Check sheet for the modelled part. Datum: model origin and axes. Units: mm. A direction names the side the tool comes from. Coordinates: 2 decimals unless noted, no trailing zeros. Loops run counter-clockwise (first coordinate to the right, second up) from the corner with the lowest first, then second, coordinate; pieces in that order, holes last. Notation, with made-up numbers: M 81.5,48 L 85.5,48 A13 cw 85.5,60 Z; hole C 58.25,27.5 d8. An arc over 180 degrees is marked long. Answer in a Markdown table with one row per item. Add a question column.
```python
from build123d import *

# Parameters (mm, degrees)
F0_R     = 14
F0_R_2   = 1.1
F1_DEPTH = 8
F3_DEPTH = 8.001
F6_R     = 0.875
F7_DEPTH = 19.125355653


# Not quite as in the source:
# - a pattern or mirror of a feature is missing from the dataset's text; its kind, count and spacing are read off the source's solid


with BuildPart() as f1:
    # F0 (on Front) → F1 (new body)
    with BuildSketch(Plane.XZ):
        Circle(F0_R)
        with Locations((-8.6602540378, -5)):
            Circle(F0_R_2, mode=Mode.SUBTRACT)
        with Locations((8.6602540378, -5)):
            Circle(F0_R_2, mode=Mode.SUBTRACT)
        with Locations((0, 10)):
            Circle(F0_R_2, mode=Mode.SUBTRACT)
    extrude(amount=F1_DEPTH)

    # F2 (on face) → F3 (cut, through all)
    with BuildSketch(Plane.XZ.offset(8)):
        with BuildLine():
            Line((-1.5, -1.3228756555), (1.5, -1.3228756555))
            ThreePointArc((1.5, -1.3228756555), (0, 2), (-1.5, -1.3228756555))
        make_face()
    extrude(amount=-F3_DEPTH, mode=Mode.SUBTRACT)

    # F6 (on line) → F7 (cut, through all)
    with BuildSketch(Plane(origin=(0, 0, 0), x_dir=(0, 1, 0), z_dir=(0.8660254038, 0, -0.5))):
        with Locations((-4, 0)):
            Circle(F6_R)
    f7 = extrude(amount=-F7_DEPTH, mode=Mode.SUBTRACT)

    # F7_copies: F7 across plane
    add(f7.mirror(Plane(origin=(1.9e-05, 0, 0), x_dir=(-1e-06, 0, 1), z_dir=(1, 0, 1e-06))), mode=Mode.SUBTRACT)


solid = f1.part
```
Q1. Cross-section at C-C (z = -5). Record the cut outline in (x, y).
Q2. Thickness scan on L1, parallel to X at y = -6.5, z = -5.5; L2, parallel to X at y = -6.5, z = -5.25; L3, parallel to Z at x = 9.25, y = -0.5. Record the ranges inside material, lowest first.
Q3. Go/stop test with flat-tipped pins: pin 1 (1.8 mm diameter, centred on x = 0, z = 10, fed in from -Y); pin 2 (3 mm diameter, centred on y = -2, z = 9, fed in from +X); pin 3 (4 mm diameter, centred on y = -6, z = -6, fed in from +X); pin 4 (1 mm diameter, centred on y = -4.5, z = -6, fed in from +X). Record where each tip stops, or that it passes through.
Q4. Mould release check, pull along X, two halves, no side actions. Record for faces 1 (the face through (0, -4, 2)), 2 (the face through (0, 0, -3)), 3 (the face through (12.932, -3.944, -5.362)), 4 (the face through (7.56, -3.94, -4.95)): released by +X, released by -X, zero draft, split by the parting line, or undercut.
Q5. Access from +Z, -Z, +X, -X, +Y, -Y to the whole of each face (thin tool, end or side, straight path). Record for faces 5 (the face through (6.636, -3.165, 4.135)), 6 (the face through (0, -4, -1.323)).
Q6. Cross-section at B-B (y = -3.75). Record the cut outline in (x, z), plus the area to 3 significant figures.
Q7. Cross-section at D-D (z = 10.75). Record the cut outline in (x, y), plus the area to 3 significant figures.
Q8. Cross-section at A-A (x = 0). Record the cut outline in (y, z).
Answer key:
| question | item | result |
|---|---|---|
| 1 | outline | M -13.08,-8 L -9.76,-8 L -9.76,0 L -13.08,0 Z; M -7.56,-8 L 7.56,-8 L 7.56,0 L -7.56,0 Z; M 9.76,-8 L 13.08,-8 L 13.08,0 L 9.76,0 Z |
| 2 | L1 | -12.87 to -9.64, -7.68 to 7.68, 9.64 to 12.87 |
| 2 | L2 | -12.98 to -9.73, -7.59 to 7.59, 9.73 to 12.98 |
| 2 | L3 | -10.51 to -5.93, -4.07 to 10.51 |
| 3 | pin 1 | through |
| 3 | pin 2 | x = 11.82 |
| 3 | pin 3 | x = 13.42 |
| 3 | pin 4 | x = 12.87 |
| 4 | face 1 | undercut |
| 4 | face 2 | zero draft |
| 4 | face 3 | split by the parting line |
| 4 | face 4 | undercut |
| 5 | face 5 | none |
| 5 | face 6 | +Y, -Y |
| 6 | outline | M -12.52,6.26 A14 ccw long 12.52,6.26 L 1.99,0.18 A2 cw 1.5,-1.32 L -1.5,-1.32 A2 cw -1.99,0.18 Z; M -11.68,7.71 L -1.15,1.63 A2 cw 1.15,1.63 L 11.68,7.71 A14 ccw Z; hole C -8.66,-5 d2.2; hole C 0,10 d2.2; hole C 8.66,-5 d2.2 |
| 6 | area | 553 mm^2 |
| 7 | outline | M -8.97,-8 L -0.8,-8 L -0.8,0 L -8.97,0 Z; M 0.8,-8 L 8.97,-8 L 8.97,0 L 0.8,0 Z |
| 7 | area | 131 mm^2 |
| 8 | outline | M -8,-14 L 0,-14 L 0,-1.32 L -8,-1.32 Z; M -8,2 L 0,2 L 0,8.9 L -8,8.9 Z; M -8,11.1 L 0,11.1 L 0,14 L -8,14 Z |
